The figure shows three views and two pictorial views of one solid part (mm, origin at its lowest corner). Answer the questions. Coordinates: 2 decimals unless noted, no trailing zeros. Write each loop counter-clockwise with the first axis right and the second up, starting at its lowest first coordinate (ties: lowest second). Pieces come first, ordered by that corner, then holes. Notation, with made-up numbers: (36.25, -22) - (53.25, -22) arc R29 ccw to (53.25, 4) - close; hole circle Ø8 at (11.5, -16). An arc over 180 degrees is marked (long way). Use a Markdown table: item, result. Add a question column.
(1) Find the intervals of material crossed by line 1 (Y direction, x = 165, z = 3.25); line 2 (Y direction, x = 12, z = 12.25); line 3 (X direction, y = 52.5, z = 12), in increasing order. Write a range as from..to.
(2) The part is cut by section A-A, the plane y = 135.25. Give the vertices of the cut face in (x, z), then the cut area to 3 significant figures.
(3) The part is cut by section C-C, the plane x = 203. Give the vertices of the cut face in (y, z).
(4) The part is cut by section B-B, the plane x = 12. Give the vertices of the cut face in (y, z).
(5) The part is cut by section D-D, the plane z = 11. Give the vertices of the cut face in (x, y), then the cut area to 3 significant figures.
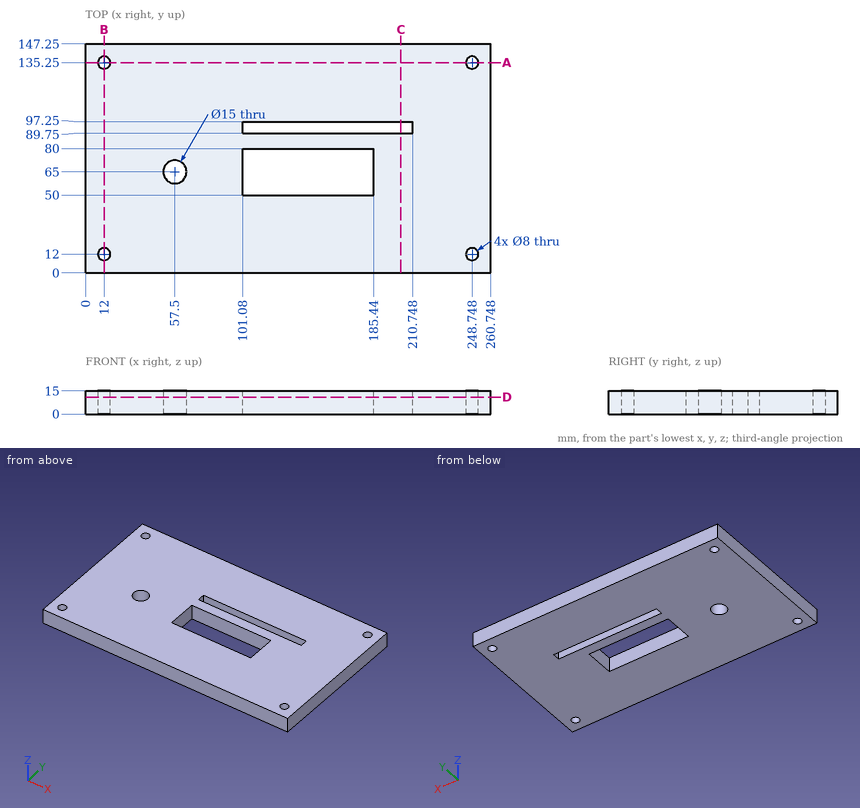
Model answer:
| question | item | result |
|---|---|---|
| 1 | line 1 | 0..50, 80..89.75, 97.25..147.25 |
| 1 | line 2 | 0..8, 16..131.25, 139.25..147.25 |
| 1 | line 3 | 0..101.08, 185.44..260.75 |
| 2 | outline | (0, 0) - (8, 0) - (8, 15) - (0, 15) - close; (16, 0) - (244.75, 0) - (244.75, 15) - (16, 15) - close; (252.75, 0) - (260.75, 0) - (260.75, 15) - (252.75, 15) - close |
| 2 | area | 3,670 mm^2 |
| 3 | outline | (0, 0) - (89.75, 0) - (89.75, 15) - (0, 15) - close; (97.25, 0) - (147.25, 0) - (147.25, 15) - (97.25, 15) - close |
| 4 | outline | (0, 0) - (8, 0) - (8, 15) - (0, 15) - close; (16, 0) - (131.25, 0) - (131.25, 15) - (16, 15) - close; (139.25, 0) - (147.25, 0) - (147.25, 15) - (139.25, 15) - close |
| 5 | outline | (0, 0) - (260.75, 0) - (260.75, 147.25) - (0, 147.25) - close; hole circle Ø8 at (12, 12); hole circle Ø8 at (12, 135.25); hole circle Ø15 at (57.5, 65); hole (101.08, 50) - (185.44, 50) - (185.44, 80) - (101.08, 80) - close; hole (101.08, 89.75) - (210.75, 89.75) - (210.75, 97.25) - (101.08, 97.25) - close; hole circle Ø8 at (248.75, 12); hole circle Ø8 at (248.75, 135.25) |
| 5 | area | 34,700 mm^2 |
